from build123d import *

# Parameters (mm, degrees)
F0_R     = 25
F1_DEPTH = 40
F2_R     = 20
F3_DEPTH = 18
F4_SIZE  = 1
F5_R     = 25
F6_DEPTH = 100
F7_SIZE  = 1
F8_R     = 26.24
F9_DEPTH = 100
F10_SIZE = 1


with BuildPart() as f1:
    # F0 (on Front) → F1 (new body)
    with BuildSketch(Plane.XZ):
        Circle(F0_R)
    extrude(amount=F1_DEPTH)

    # F2 (on face) → F3 (join)
    with BuildSketch(Plane.XZ.offset(40)):
        Circle(F2_R)
    extrude(amount=F3_DEPTH)

    # F4
    f4_edges = [f1.edges().sort_by_distance(p)[0] for p in [
        (-25, -40, 0),
        (-25, 0, 0),
    ]]
    chamfer(f4_edges, length=F4_SIZE)

    # F5 (on face) → F6 (join)
    with BuildSketch(Plane.XZ.offset(58)):
        Circle(F5_R)
    extrude(amount=F6_DEPTH)

    # F7
    f7_edges = [f1.edges().sort_by_distance(p)[0] for p in [
        (-25, -58, 0),
    ]]
    chamfer(f7_edges, length=F7_SIZE)

    # F8 (on face) → F9 (join)
    with BuildSketch(Plane.XZ.offset(158)):
        Circle(F8_R)
    extrude(amount=F9_DEPTH)

    # F10
    f10_edges = [f1.edges().sort_by_distance(p)[0] for p in [
        (-26.24, -258, 0),
    ]]
    chamfer(f10_edges, length=F10_SIZE)


solid = f1.part
For this review, take the finished solid that the model builds, in its own axes (mm). A direction names the side the tool comes from. Round coordinates to 2 decimals unless told otherwise and drop trailing zeros. Order: outer loops, then holes, each group sorted by start corner. A loop starts at its lowest first (then second) coordinate and runs counter-clockwise, first axis right, second up. Notation, with made-up numbers: (-28, 25.25) -> (-1, 25.25) arc R18 cw to (-1, 38.25) -> close; hole circle Ø11 at (22, 21). An arc over 180 degrees is marked (long way). Put each result on its own line as item: value.
Q1. Machinability: for faces 1 (the cylindrical face through (23.846, -107.807, 7.509)), 2 (the flat face through (-5, -58, 20)), 3 (the flat face through (0, -258, 0)), which of the approach directions +Z, -Z, +X, -X, +Y, -Y give a long, thin tool a straight path to every point of the face, cutting with its end or side? Answer none if there is none.
Check result:
face 1: +Y
face 2: none
face 3: +Z, -Z, +X, -X, -Y
Q2. Add section C-C on y = -178. Write out the cut boundary in (x, z).
Check result:
outline: circle Ø52.48 at (0, 0)
Q3. Add section D-D on y = -120. Write out the cut boundary in (x, z).
Check result:
outline: circle Ø50 at (0, 0)
Q4. Add section A-A on z = 0. Write out the cut boundary in (x, y), plus the area to 3 significant figures.
Check result:
outline: (-26.24, -257) -> (-25.24, -258) -> (25.24, -258) -> (26.24, -257) -> (26.24, -158) -> (25, -158) -> (25, -59) -> (24, -58) -> (20, -58) -> (20, -40) -> (24, -40) -> (25, -39) -> (25, -1) -> (24, 0) -> (-24, 0) -> (-25, -1) -> (-25, -39) -> (-24, -40) -> (-20, -40) -> (-20, -58) -> (-24, -58) -> (-25, -59) -> (-25, -158) -> (-26.24, -158) -> close
area: 13,000 mm2
Q5. Insertion check: pin 1 Ø10 at (y, z) = (-210, -20.5) entering from +X; pin 2 Ø2 at (x, y) = (-21, -158) entering from -Z; pin 3 Ø5 at (y, z) = (-162, 18) entering from -X. Each pin has a flat end and moves straight along its axis. Give the tip position at first contact, or say it passes through.
Check result:
pin 1: x = 21.17
pin 2: z = -16.99
pin 3: x = -21.17
Q6. Add section B-B on x = 0. Write out the cut boundary in (y, z).
Check result:
outline: (-258, -25.24) -> (-257, -26.24) -> (-158, -26.24) -> (-158, -25) -> (-59, -25) -> (-58, -24) -> (-58, -20) -> (-40, -20) -> (-40, -24) -> (-39, -25) -> (-1, -25) -> (0, -24) -> (0, 24) -> (-1, 25) -> (-39, 25) -> (-40, 24) -> (-40, 20) -> (-58, 20) -> (-58, 24) -> (-59, 25) -> (-158, 25) -> (-158, 26.24) -> (-257, 26.24) -> (-258, 25.24) -> close
Q7. For probe 1 along Y at (x, z) = (10.5, 19.5); probe 2 along X at (y, z) = (-201.5, -8); probe 3 along Z at (x, y) = (-1, -215), list the stretches that pass through material, from the lowest coordinate up. Write a range as [from, to].
Check result:
probe 1: [-258, -58], [-40, 0]
probe 2: [-24.99, 24.99]
probe 3: [-26.22, 26.22]
Q8. Mouldability with a two-part tool opening along Y and no side actions: class faces 4 (the cylindrical face through (23.846, -19.734, 7.509)), 5 (the flat face through (13.5, -158, -21.3)), 6 (the flat face through (-5, -40, 20)) as pulls with the +Y half, pulls with the -Y half, needs draft (parallel to the pull), parting line crosses it, or undercut.
Check result:
face 4: needs draft
face 5: pulls with the +Y half
face 6: undercut
